```python
from build123d import *

# Parameters (mm, degrees)
F0_W     = 14
F0_H     = 111.6
F1_DEPTH = 3
F2_W     = 1
F2_H     = 111.6
F3_DEPTH = 0.5
F4_R     = 1.5
F5_DEPTH = 25


with BuildPart() as f1:
    # F0 (on Top) → F1 (new body)
    with BuildSketch(Plane.XY):
        with Locations((7, 55.8)):
            Rectangle(F0_W, F0_H)
    extrude(amount=F1_DEPTH)

    # F2 (on face) → F3 (join)
    with BuildSketch(Plane.XY.offset(3)):
        with Locations((0.5, 55.8)):
            Rectangle(F2_W, F2_H)
        with Locations((13.5, 55.8)):
            Rectangle(F2_W, F2_H)
    extrude(amount=F3_DEPTH)

    # F4 (on face) → F5 (cut)
    with BuildSketch(Plane.XY.offset(3)):
        with BuildLine():
            Line((5.5, 14.5), (5.5, 4.5))
            ThreePointArc((5.5, 4.5), (7, 3), (8.5, 4.5))
            Line((8.5, 4.5), (8.5, 14.5))
            ThreePointArc((8.5, 14.5), (7, 16), (5.5, 14.5))
        make_face()
        with Locations((7, 24.5)):
            Circle(F4_R)
        with Locations((7, 34.5)):
            Circle(F4_R)
        with Locations((7, 44.5)):
            Circle(F4_R)
        with Locations((7, 54.5)):
            Circle(F4_R)
        with BuildLine():
            Line((5.5, 74.5), (5.5, 64.5))
            ThreePointArc((5.5, 64.5), (7, 63), (8.5, 64.5))
            Line((8.5, 64.5), (8.5, 74.5))
            ThreePointArc((8.5, 74.5), (7, 76), (5.5, 74.5))
        make_face()
        with Locations((7, 84.5)):
            Circle(F4_R)
        with Locations((7, 94.5)):
            Circle(F4_R)
        with Locations((7, 104.5)):
            Circle(F4_R)
    extrude(amount=-F5_DEPTH, mode=Mode.SUBTRACT)


solid = f1.part
```
Here's how the part is built. I have some questions about the finished solid (model axes, mm). A direction names the side the tool comes from. Round coordinates to 2 decimals unless told otherwise and drop trailing zeros. Write each loop counter-clockwise with the first axis right and the second up, starting at its lowest first coordinate (ties: lowest second). Pieces come first, ordered by that corner, then holes.
Q1. If we section it at C-C on x = 4: Write out the boundary of the cut face in (y, z).
Q2. Which directions (+Z, -Z, +X, -X, +Y, -Y) give clear straight access to the entire face, cutting with the end or side of a thin tool? Please do faces 1 (the flat face through (7, 57, 0)), 2 (the flat face through (7, 57, 3)), 3 (the cylindrical face through (7, 63, 2)).
Q3. Will this pin go through, and if not, where does the flat tip stop? P1, Ø3.5, axis at x = 7.5, y = 73.5, coming from the +Z side.
Q4. Please list where these lines run through material, in increasing order: probe 1 along X at (y, z) = (94.5, 0.95); probe 2 along Z at (x, y) = (8.5, 85.5); probe 3 along X at (y, z) = (95.5, 1).
Q5. If we mould it in two halves opening along X, with no side actions, what happens to faces 4 (the flat face through (7, 111.6, 2)), 5 (the flat face through (8.5, 9, 2)), 6 (the flat face through (14, 55, 2))? For each: +X half, -X half, draft (parallel to the pull), parting line (faces both ways), or undercut.
Q6. If we section it at A-A on y = 54.5: Write out the boundary of the cut face in (x, z), plus the area to 3 significant figures.
Q7. If we section it at B-B on z = 0.85: Give the number of separate pieces and of enclosed holes in the cut face, plus the area to 3 significant figures.
Answer below:
1. outline: (0, 0) - (111.6, 0) - (111.6, 3) - (0, 3) - close
2. face 1: -Z, +X, -X, +Y, -Y
2. face 2: +Z, +Y, -Y
2. face 3: +Z, -Z
3. P1: stops at z = 3
4. probe 1: x = 0 to 5.5, 8.5 to 14
4. probe 2: z = 0 to 3
4. probe 3: x = 0 to 5.88, 8.12 to 14
5. face 4: draft
5. face 5: undercut
5. face 6: +X half
6. outline: (0, 0) - (5.5, 0) - (5.5, 3) - (1, 3) - (1, 3.5) - (0, 3.5) - close; (8.5, 0) - (14, 0) - (14, 3.5) - (13, 3.5) - (13, 3) - (8.5, 3) - close
6. area: 34.0 mm2
7. separate pieces: 1
7. enclosed holes: 9
7. area: 1,440 mm2
